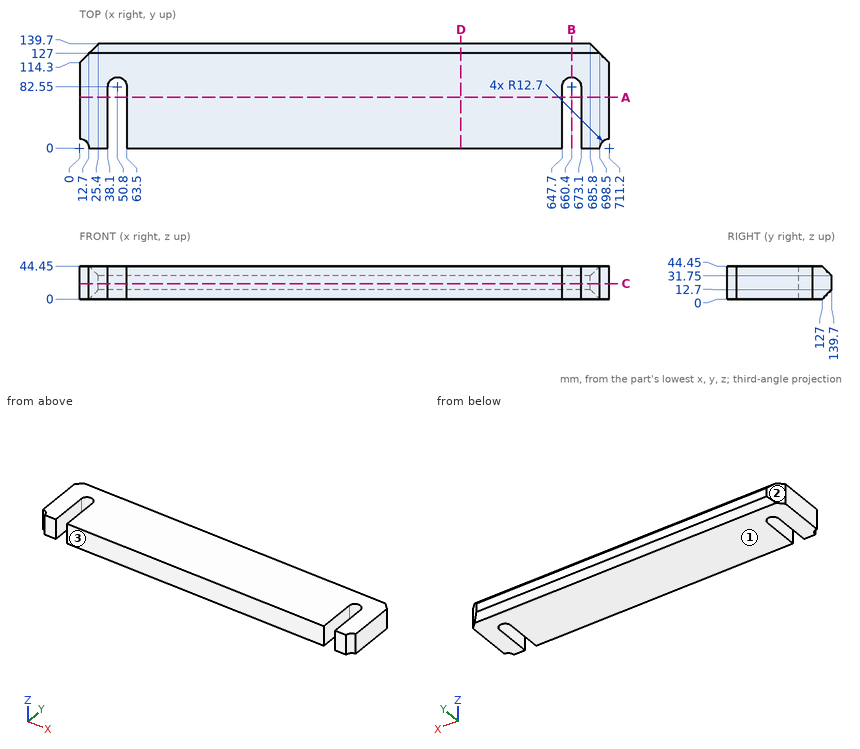
Print and shaded views of the part. All mm, measured from the part's lowest x, y and z. Give positions to 0.01 mm unless a question says otherwise; leave off trailing zeros. Order: outer loops, then holes, each group sorted by start corner. A loop starts at its lowest first (then second) coordinate and runs counter-clockwise, first axis right, second up. Notation, with made-up numbers: (62.5, 56.25) - (87.5, 56.25) arc R19 ccw to (87.5, 90.25) - close; hole circle Ø10 at (47, 58). An arc over 180 degrees is marked (long way). One line per item, written item: value.
Item 1: Pin check, flat tip, straight feed: pin 1 Ø4 at (y, z) = (122, 26) entering from -X. Stop position of the tip, or through.
Response values:
pin 1: x = 5.7
Item 2: Slice it at D-D (x = 512). List the corners of the cut face in (y, z).
Response values:
outline: (0, 0) - (127, 0) - (139.7, 12.7) - (139.7, 31.75) - (127, 44.45) - (0, 44.45) - close
Item 3: Wall check: line 1 (X direction, y = 37.5, z = 14.5); line 2 (X direction, y = 86.5, z = 33); line 3 (Z direction, x = 371, y = 128). Give the ranges that are in metal, low to high.
Response values:
line 1: 0 to 38.1, 63.5 to 647.7, 673.1 to 711.2
line 2: 0 to 38.73, 62.87 to 648.33, 672.47 to 711.2
line 3: 1 to 43.45
Item 4: Slice it at A-A (y = 68). List the corners of the cut face in (x, z).
Response values:
outline: (0, 0) - (38.1, 0) - (38.1, 44.45) - (0, 44.45) - close; (63.5, 0) - (647.7, 0) - (647.7, 44.45) - (63.5, 44.45) - close; (673.1, 0) - (711.2, 0) - (711.2, 44.45) - (673.1, 44.45) - close
Item 5: Two-plate mould, pull along Y, no slides. Class the marked faces 1, 2 and 3: released by +Y, released by -Y, zero draft, split by the parting line, or undercut.
Response values:
face 1: zero draft
face 2: released by +Y
face 3: released by -Y
Item 6: Slice it at C-C (z = 21). List the corners of the cut face in (x, y), then the cut area to 3 significant figures.
Response values:
outline: (0, 12.7) arc R12.7 cw to (12.7, 0) - (38.1, 0) - (38.1, 82.55) arc R12.7 cw to (63.5, 82.55) - (63.5, 0) - (647.7, 0) - (647.7, 82.55) arc R12.7 cw to (673.1, 82.55) - (673.1, 0) - (698.5, 0) arc R12.7 cw to (711.2, 12.7) - (711.2, 114.3) - (685.8, 139.7) - (25.4, 139.7) - (0, 114.3) - close
area: 93,800 mm2
Item 7: Slice it at B-B (x = 660.4). List the corners of the cut face in (y, z).
Response values:
outline: (95.25, 0) - (127, 0) - (139.7, 12.7) - (139.7, 31.75) - (127, 44.45) - (95.25, 44.45) - close
